The listing builds one solid part. Answer for the finished solid, in the listing's coordinates (mm). Face numbers are marked on the shaded views. Round coordinates to 2 decimals unless told otherwise and drop trailing zeros. Loops run counter-clockwise (first coordinate to the right, second up) from the corner with the lowest first, then second, coordinate; pieces in that order, holes last. Notation, with made-up numbers: (-27.75, -25) -> (-21.75, -25) arc R11 cw to (-21.75, -20) -> close; hole circle Ø5 at (41.25, 63). An arc over 180 degrees is marked (long way). Use a Markdown table: item, result. Add a question column.
Q1. Given pin 1 Ø1.2 at (x, y) = (14.5, 14) entering from +Z; pin 2 Ø8 at (x, z) = (-36.5, 5) entering from +Y; pin 3 Ø2.5 at (x, z) = (22, 11.5) entering from -Y, each flat-ended and moving along its own axis, determine where each tip first touches the part or whether it passes through.
Q2. Section A-A on z = 11.5 is taken. Give the vertices of the cut face in (x, y).
Q3. For a pull along Y with two mould halves and no side action, classify the marked faces 1, 2 and 3 as released by +Y, released by -Y, zero draft, split by the parting line, or undercut.
Q4. Section B-B on x = 0 is taken. Give the vertices of the cut face in (y, z).
Q5. Section C-C on y = -6 is taken. Give the vertices of the cut face in (x, z), then the cut area to 3 significant figures.
Q6. Consider line 1 (X direction, y = 28.5, z = 4); line 2 (Y direction, x = 10, z = 5.5); line 3 (Z direction, x = -34.5, y = -10). Determine where each line is inside the solid, lowest interval first.
Autodesk Inventor part; units mm, degrees
ref_plane "YZ Plane" through (0, 0, 0) normal (1, 0, 0) x (0, 1, 0)
ref_plane "XZ Plane" through (0, 0, 0) normal (0, 1, 0) x (-1, 0, 0)
ref_plane "XY Plane" through (0, 0, 0) normal (0, 0, 1) x (1, 0, 0)
sketch "スケッチ1" plane through (0, 0, 0) normal (0, 0, 1) x (1, 0, 0)
  circle A0 centre (0, 0) radius 50
  circle A1 centre (0, 0) radius 40
  circle A2 centre (-33.4581, 30.0925) radius 2.05
  circle A3 centre (-9.3318, -44.0218) radius 2.05
  circle A4 centre (42.7899, 13.9293) radius 2.05
  dimension "d0" = 100
  dimension "d1" = 80
  dimension "d2" = 4.1
  dimension "d4" = 45
  dimension "d7" = 360
extrude "押し出し1" add sketch "スケッチ1" along normal blind 10 contours A0 | A1
sketch "スケッチ2" plane through (0, 0, 0) normal (0, 0, -1) x (-1, 0, 0)
  circle A0 centre (0, 0) radius 50
  circle A1 centre (0, 0) radius 40
  circle A2 centre (-33.4581, 30.0925) radius 2.05
  circle A3 centre (-9.3318, -44.0218) radius 2.05
  circle A4 centre (42.7899, 13.9293) radius 2.05
  dimension "d13" = 100
  dimension "d14" = 80
  dimension "d17" = 360
extrude "押し出し2" cut sketch "スケッチ2" against normal blind 5 contours A1
sketch "スケッチ3" plane through (0, 0, 5) normal (0, 0, -1) x (-1, 0, 0)
  circle A0 centre (0, 0) radius 41
  circle A1 centre (0, 0) radius 40
  dimension "d21" = 80
  dimension "d22" = 82
extrude "押し出し3" cut sketch "スケッチ3" along normal blind 2
sketch "スケッチ4" plane through (0, 0, 5) normal (0, 0, -1) x (-1, 0, 0)
  circle A0 centre (0, 0) radius 35
  circle A1 centre (0, 0) radius 16
  dimension "d27" = 70
  dimension "d28" = 32
extrude "押し出し4" cut sketch "スケッチ4" against normal blind 1.5
sketch "スケッチ5" plane through (0, 0, 5) normal (0, 0, -1) x (-1, 0, 0)
  circle A0 centre (0, 0) radius 11
  dimension "d31" = 22
extrude "押し出し5" cut sketch "スケッチ5" against normal blind 5
sketch "スケッチ8" plane through (0, 0, 10) normal (0, 0, 1) x (1, 0, 0)
  circle A0 centre (0, 0) radius 11
  line L0 (0, 0) -> (3.5, 0)
  line L1 (11.5, 10) -> (11.5, 15)
  line L2 (11.5, 15) -> (26, 15)
  line L3 (11.5, 10) -> (26, 10)
  line L4 (26, 10) -> (26, 15)
  circle A1 centre (14.75, 13.5) radius 1.25
  circle A2 centre (22.75, 13.5) radius 1.25
  line L5 (-70, 0) -> (70, 0)
  line L6 (11.5, -10) -> (11.5, -15)
  line L7 (11.5, -15) -> (26, -15)
  line L8 (11.5, -10) -> (26, -10)
  line L9 (26, -10) -> (26, -15)
  circle A3 centre (14.75, -13.5) radius 1.25
  circle A4 centre (22.75, -13.5) radius 1.25
  line L10 (0, -70) -> (0, 70)
  line L11 (-98, 0) -> (98, 0)
  dimension "d54" = 5
  dimension "d55" = 14.5
  dimension "d56" = 2.5
  dimension "d57" = 3.25
  dimension "d58" = 1.5
  dimension "d59" = 2.5
  dimension "d60" = 3.25
  dimension "d64" = 27
  dimension "d65" = 11.5
extrude "押し出し7" add sketch "スケッチ8" along normal blind 5 contours L1 L2 L4 L3 | L8 L9 L7 L6
properties part number "rotate_plate_3"
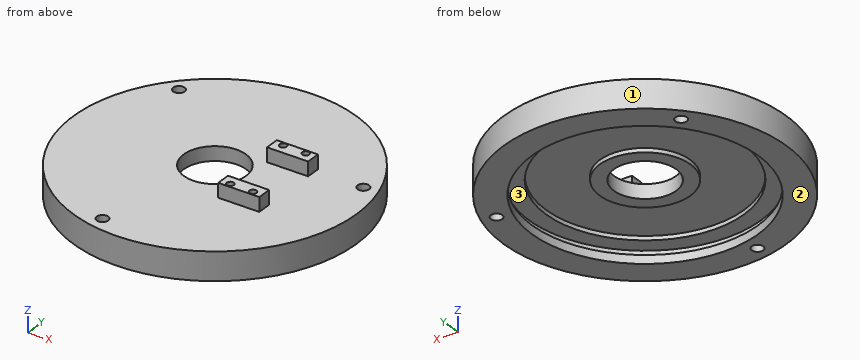
Checked values:
| question | item | result |
|---|---|---|
| 1 | pin 1 | stops at z = 10 |
| 1 | pin 2 | stops at y = 38 |
| 1 | pin 3 | stops at y = -15 |
| 2 | outline | (11.5, -15) -> (26, -15) -> (26, -10) -> (11.5, -10) -> close; (11.5, 10) -> (26, 10) -> (26, 15) -> (11.5, 15) -> close; hole circle Ø2.5 at (14.75, -13.5); hole circle Ø2.5 at (14.75, 13.5); hole circle Ø2.5 at (22.75, -13.5); hole circle Ø2.5 at (22.75, 13.5) |
| 3 | face 1 | split by the parting line |
| 3 | face 2 | zero draft |
| 3 | face 3 | undercut |
| 4 | outline | (-50, 0) -> (-40, 0) -> (-40, 3) -> (-41, 3) -> (-41, 5) -> (-35, 5) -> (-35, 6.5) -> (-16, 6.5) -> (-16, 5) -> (-11, 5) -> (-11, 10) -> (-50, 10) -> close; (11, 5) -> (16, 5) -> (16, 6.5) -> (35, 6.5) -> (35, 5) -> (41, 5) -> (41, 3) -> (40, 3) -> (40, 0) -> (50, 0) -> (50, 10) -> (11, 10) -> close |
| 5 | outline | (-49.64, 0) -> (-39.55, 0) -> (-39.55, 3) -> (-40.56, 3) -> (-40.56, 5) -> (-34.48, 5) -> (-34.48, 6.5) -> (-14.83, 6.5) -> (-14.83, 5) -> (-9.22, 5) -> (-9.22, 10) -> (-49.64, 10) -> close; (9.22, 5) -> (14.83, 5) -> (14.83, 6.5) -> (34.48, 6.5) -> (34.48, 5) -> (40.56, 5) -> (40.56, 3) -> (39.55, 3) -> (39.55, 0) -> (49.64, 0) -> (49.64, 10) -> (9.22, 10) -> close |
| 5 | area | 442 mm2 |
| 6 | line 1 | x = -41.08 to -34.75, -32.17 to -29.47, 29.47 to 41.08 |
| 6 | line 2 | y = -48.99 to -33.54, -12.49 to -4.58, 4.58 to 12.49, 33.54 to 48.99 |
| 6 | line 3 | z = 5 to 10 |
